Can you work these out from the model? Positions are in its coordinate system, mm. A direction names the side the tool comes from. Coordinates: 2 decimals unless noted, no trailing zeros. Loops run counter-clockwise (first coordinate to the right, second up) from the corner with the lowest first, then second, coordinate; pieces in that order, holes last. Notation, with made-up numbers: (20.5, 16) -> (76.5, 16) arc R12 cw to (76.5, 28) -> close; hole circle Ø7 at (-10, 89). An arc over 180 degrees is marked (long way). Put each result on its own line as item: value. Start each with the question number.
Item 1: If we section it at D-D on z = 5: Please give me the cut outline in (x, y), plus the area to 3 significant figures.
Item 2: Will these pins go through, and if not, where does the flat tip stop? P1, Ø8, axis at x = -3.5, y = 15.5, coming from the +Z side; P2, Ø4, axis at x = -0.5, z = 6, coming from the -Y side; P3, Ø4, axis at x = -2.5, z = 7, coming from the +Y side.
Item 3: If we section it at B-B on y = 9: Please give me the cut outline in (x, z), plus the area to 3 significant figures.
Item 4: For faces 1 (the flat face through (6, -5, 2)), 2 (the cylindrical face through (-1.987, 21.544, 0.986)), which set-ups out of +Z, -Z, +X, -X, +Y, -Y let a thin tool reach every point of the face, with its end or its side?
Item 5: If we section it at A-A on x = 0: Please give me the cut outline in (y, z).
Item 6: If we section it at C-C on x = 4: Please give me the cut outline in (y, z), plus the area to 3 significant figures.
Item 7: Please list where these lines run through material, in increasing order: L1, parallel to Z at x = 3, y = 6; L2, parallel to X at y = 6.5, z = 1.25; L3, parallel to Z at x = -13.5, y = 9.5. Write a range as from..to.
```python
from build123d import *

# Parameters (mm, degrees)
F0_R     = 12.55535
F2_DEPTH = 7
F1_R     = 15.260339
F3_DEPTH = 2
F4_R     = 1.26869
F5_DEPTH = 2


with BuildPart() as f2:
    # F0 (on Top) → F2 (new body)
    with BuildSketch(Plane.XY):
        with Locations((0, 6.495178)):
            Circle(F0_R)
    extrude(amount=F2_DEPTH)

    # F1 (on Top) → F3 (join)
    with BuildSketch(Plane.XY):
        with Locations((0, 6.413349)):
            Circle(F1_R)
    extrude(amount=F3_DEPTH)

    # F4 (on face) → F5 (join)
    with BuildSketch(Plane.XY.offset(7)):
        with Locations((0, 6.495178)):
            Circle(F4_R)
    extrude(amount=F5_DEPTH)


solid = f2.part
```
Solutions:
1. outline: circle Ø25.11 at (0, 6.5)
1. area: 495 mm^2
2. P1: z = 7
2. P2: y = -6.06
2. P3: y = 19.04
3. outline: (-15.04, 0) -> (15.04, 0) -> (15.04, 2) -> (12.3, 2) -> (12.3, 7) -> (-12.3, 7) -> (-12.3, 2) -> (-15.04, 2) -> close
3. area: 183 mm^2
4. face 1: +Z
4. face 2: +Z, -Z
5. outline: (-8.85, 0) -> (21.67, 0) -> (21.67, 2) -> (19.05, 2) -> (19.05, 7) -> (7.76, 7) -> (7.76, 9) -> (5.23, 9) -> (5.23, 7) -> (-6.06, 7) -> (-6.06, 2) -> (-8.85, 2) -> close
6. outline: (-8.31, 0) -> (21.14, 0) -> (21.14, 2) -> (18.4, 2) -> (18.4, 7) -> (-5.41, 7) -> (-5.41, 2) -> (-8.31, 2) -> close
6. area: 178 mm^2
7. L1: 0..7
7. L2: -15.26..15.26
7. L3: 0..2
